Can you work these out from the model? Positions are in its coordinate system, mm. Round coordinates to 2 decimals unless told otherwise and drop trailing zeros. Write each loop counter-clockwise with the first axis right and the second up, starting at its lowest first coordinate (ties: lowest second). Pieces come first, ordered by that corner, then holes. Notation, with made-up numbers: M 64,19.25 L 88,19.25 A26 ccw 88,58.25 Z; hole C 10.5,-26.75 d6. An arc over 180 degrees is marked long. Answer as a JSON object with one key per item and string values. Group by question number.
1) Please list where these lines run through material, in increasing order: L1, parallel to X at y = 3.35, z = 0; L2, parallel to Z at x = 50.5, y = 4.75; L3, parallel to Z at x = 48, y = 4.15. Write a range as [from, to].
2) I'm going to push flat-ended pins straight in: pin 1 Ø1.5 at (y, z) = (2.5, 27.5) entering from -X; pin 2 Ø1 at (y, z) = (1.5, -49) entering from -X. Where does each tip first touch, or does it pass through?
3) Suppose I cut it at D-D, the plane y = 3.6. State how many separate pieces and enclosed holes the cut face has, and give its area (3 significant figures).
4) Suppose I cut it at B-B, the plane z = 0. Write out the boundary of the cut face in (x, y), and give its area (3 significant figures).
5) Suppose I cut it at C-C, the plane z = -19. Write out the boundary of the cut face in (x, y), and give its area (3 significant figures).
6) Suppose I cut it at A-A, the plane x = 0. Write out the boundary of the cut face in (y, z).
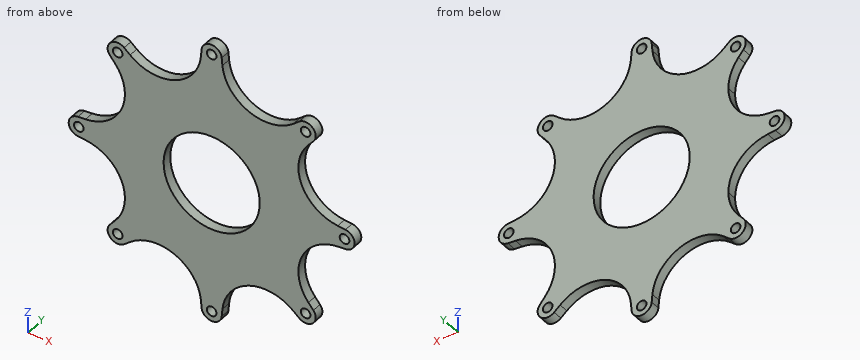
from build123d import *

# Parameters (mm, degrees)
SKETCH1_R           = 5.25
BOSS_EXTRUDE1_DEPTH = 5
SKETCH2_R           = 2.5
CUT_EXTRUDE1_DEPTH  = 10
SKETCH3_R           = 25
CUT_EXTRUDE2_DEPTH  = 10


with BuildPart() as part:
    # Sketch1 → Boss-Extrude1 (new body)
    with BuildSketch(Plane(origin=(0, 0, 0), x_dir=(1, 0, 0), z_dir=(0, 1, 0))):
        with BuildLine():
            ThreePointArc((69.572261498, -5.228532951), (63.847979746, 0), (69.572261498, 5.228532951))
            Line((69.572261498, 5.228532951), (65.565343666, 5.592001639))
            ThreePointArc((65.565343666, 5.592001639), (46.810690265, 19.389622772), (50.315841396, 42.407556838))
            Line((50.315841396, 42.407556838), (52.892148993, 45.497886783))
            ThreePointArc((52.892148993, 45.497886783), (45.147339444, 45.147339444), (45.497886783, 52.892148993))
            Line((45.497886783, 52.892148993), (42.407556838, 50.315841396))
            ThreePointArc((42.407556838, 50.315841396), (19.389622772, 46.810690265), (5.592001639, 65.565343666))
            Line((5.592001639, 65.565343666), (5.228532951, 69.572261498))
            ThreePointArc((5.228532951, 69.572261498), (5.244630492, 69.33536341), (5.25, 69.097979746))
            ThreePointArc((5.25, 69.097979746), (-0.237383663, 63.853349255), (-5.228532951, 69.572261498))
            Line((-5.228532951, 69.572261498), (-5.592001639, 65.565343666))
            ThreePointArc((-5.592001639, 65.565343666), (-19.389622772, 46.810690265), (-42.407556838, 50.315841396))
            Line((-42.407556838, 50.315841396), (-45.497886783, 52.892148993))
            ThreePointArc((-45.497886783, 52.892148993), (-44.105086073, 51.085997151), (-43.609650045, 48.859650045))
            ThreePointArc((-43.609650045, 48.859650045), (-47.071930755, 43.923400483), (-52.892148993, 45.497886783))
            Line((-52.892148993, 45.497886783), (-50.315841396, 42.407556838))
            ThreePointArc((-50.315841396, 42.407556838), (-46.44262448, 35.661654101), (-45.097979746, 28))
            ThreePointArc((-45.097979746, 28), (-50.984968102, 12.825750625), (-65.565343666, 5.592001639))
            Line((-65.565343666, 5.592001639), (-69.572261498, 5.228532951))
            ThreePointArc((-69.572261498, 5.228532951), (-65.557321559, 3.876369384), (-63.847979746, 0))
            ThreePointArc((-63.847979746, 0), (-65.557321559, -3.876369384), (-69.572261498, -5.228532951))
            Line((-69.572261498, -5.228532951), (-65.565343666, -5.592001639))
            ThreePointArc((-65.565343666, -5.592001639), (-50.984968102, -12.825750625), (-45.097979746, -28))
            ThreePointArc((-45.097979746, -28), (-46.44262448, -35.661654101), (-50.315841396, -42.407556838))
            Line((-50.315841396, -42.407556838), (-52.892148993, -45.497886783))
            ThreePointArc((-52.892148993, -45.497886783), (-47.071930755, -43.923400483), (-43.609650045, -48.859650045))
            ThreePointArc((-43.609650045, -48.859650045), (-44.105086073, -51.085997151), (-45.497886783, -52.892148993))
            Line((-45.497886783, -52.892148993), (-42.407556838, -50.315841396))
            ThreePointArc((-42.407556838, -50.315841396), (-19.389622772, -46.810690265), (-5.592001639, -65.565343666))
            Line((-5.592001639, -65.565343666), (-5.228532951, -69.572261498))
            ThreePointArc((-5.228532951, -69.572261498), (-0.237383663, -63.853349255), (5.25, -69.097979746))
            ThreePointArc((5.25, -69.097979746), (5.244630492, -69.33536341), (5.228532951, -69.572261498))
            Line((5.228532951, -69.572261498), (5.592001639, -65.565343666))
            ThreePointArc((5.592001639, -65.565343666), (19.389622772, -46.810690265), (42.407556838, -50.315841396))
            Line((42.407556838, -50.315841396), (45.497886783, -52.892148993))
            ThreePointArc((45.497886783, -52.892148993), (45.147339444, -45.147339444), (52.892148993, -45.497886783))
            Line((52.892148993, -45.497886783), (50.315841396, -42.407556838))
            ThreePointArc((50.315841396, -42.407556838), (46.810690265, -19.389622772), (65.565343666, -5.592001639))
            Line((65.565343666, -5.592001639), (69.572261498, -5.228532951))
        make_face()
        with Locations((0, -69.097979746)):
            Circle(SKETCH1_R)
        with Locations((48.859650045, -48.859650045)):
            Circle(SKETCH1_R)
        with Locations((69.097979746, 0)):
            Circle(SKETCH1_R)
        with Locations((48.859650045, 48.859650045)):
            Circle(SKETCH1_R)
        with Locations((-48.859650045, -48.859650045)):
            Circle(SKETCH1_R)
        with Locations((-69.097979746, 0)):
            Circle(SKETCH1_R)
        with Locations((-48.859650045, 48.859650045)):
            Circle(SKETCH1_R)
        with Locations((0, 69.097979746)):
            Circle(SKETCH1_R)
    extrude(amount=BOSS_EXTRUDE1_DEPTH)

    # Sketch2 → Cut-Extrude1 (cut)
    with BuildSketch(Plane(origin=(0, 5, 0), x_dir=(1, 0, 0), z_dir=(0, 1, 0))):
        with Locations(Location((69.097979746, 0, 0), (0, 0, 270))):
            Circle(SKETCH2_R)
        with Locations(Location((48.859650045, -48.859650045, 0), (0, 0, 270))):
            Circle(SKETCH2_R)
        with Locations(Location((0, -69.097979746, 0), (0, 0, 270))):
            Circle(SKETCH2_R)
        with Locations(Location((-48.859650045, -48.859650045, 0), (0, 0, 270))):
            Circle(SKETCH2_R)
        with Locations(Location((-69.097979746, 0, 0), (0, 0, 270))):
            Circle(SKETCH2_R)
        with Locations(Location((-48.859650045, 48.859650045, 0), (0, 0, 270))):
            Circle(SKETCH2_R)
        with Locations(Location((0, 69.097979746, 0), (0, 0, 270))):
            Circle(SKETCH2_R)
        with Locations(Location((48.859650045, 48.859650045, 0), (0, 0, 270))):
            Circle(SKETCH2_R)
    extrude(amount=-CUT_EXTRUDE1_DEPTH, mode=Mode.SUBTRACT)

    # Sketch3 → Cut-Extrude2 (cut)
    with BuildSketch(Plane(origin=(0, 5, 0), x_dir=(1, 0, 0), z_dir=(0, 1, 0))):
        with Locations(Location((0, 0, 0), (0, 0, 270))):
            Circle(SKETCH3_R)
    extrude(amount=-CUT_EXTRUDE2_DEPTH, mode=Mode.SUBTRACT)


solid = part.part
Results:
{
 "1": {"L1": "[-74.35, -71.6], [-66.6, -25], [25, 66.6], [71.6, 74.35]", "L2": "[-53.85, -50.75], [-46.97, -42.63], [-13.37, 13.37], [42.63, 46.97], [50.75, 53.85]", "L3": "[-54.04, -51.21], [-46.51, -39.05], [-16.95, 16.95], [39.05, 46.51], [51.21, 54.04]"},
 "2": {"pin 1": "x = -45.13", "pin 2": "x = -54.11"},
 "3": {"separate pieces": "1", "enclosed holes": "9", "area": "8,720 mm^2"},
 "4": {"outline": "M -74.35,0 L -71.6,0 L -71.6,5 L -74.35,5 Z; M -66.6,0 L -25,0 L -25,5 L -66.6,5 Z; M 25,0 L 66.6,0 L 66.6,5 L 25,5 Z; M 71.6,0 L 74.35,0 L 74.35,5 L 71.6,5 Z", "area": "443 mm^2"},
 "5": {"outline": "M -46.98,0 L -16.25,0 L -16.25,5 L -46.98,5 Z; M 16.25,0 L 46.98,0 L 46.98,5 L 16.25,5 Z", "area": "307 mm^2"},
 "6": {"outline": "M 0,-74.35 L 5,-74.35 L 5,-71.6 L 0,-71.6 Z; M 0,-66.6 L 5,-66.6 L 5,-25 L 0,-25 Z; M 0,25 L 5,25 L 5,66.6 L 0,66.6 Z; M 0,71.6 L 5,71.6 L 5,74.35 L 0,74.35 Z"}
}
